Work out the finished part from the listing and answer in its coordinate system (mm). Face numbers are marked on the shaded views. A direction names the side the tool comes from. Coordinates: 2 decimals unless noted, no trailing zeros. Order: outer loops, then holes, each group sorted by start corner. A loop starts at its lowest first (then second) coordinate and runs counter-clockwise, first axis right, second up. Notation, with made-up numbers: (10, -20) -> (55, -20) arc R32 ccw to (55, 17) -> close; hole circle Ø5 at (0, 57.5). An arc over 180 degrees is marked (long way). Answer as CSV lines item,"result". Start each with the question number.
Item 1: Section C-C (x = 10) is taken. Write down the section's boundary in (y, z), then the cut area to 3 significant figures.
Item 2: Which of the six approach directions +Z, -Z, +X, -X, +Y, -Y give full straight-line access (tool end or side, diameter ignored) to the marked faces 4, 5 and 6?
Item 3: Straight lines are drawn through the part: L1, parallel to Z at x = 11.8, y = 0; L2, parallel to Y at x = 2.25, z = 7.75; L3, parallel to Z at x = 8, y = -5. For each, find the intervals that lie inside material, in ascending order.
Item 4: For a pull along X with two mould halves and no side action, classify the marked faces 1, 2 and 3 as pulls with the +X half, pulls with the -X half, needs draft (parallel to the pull), parting line crosses it, or undercut.
Item 5: Section B-B (y = 3.75) is taken. Write down the section's boundary in (x, z), then the cut area to 3 significant figures.
Item 6: Section A-A (x = 0) is taken. Write down the section's boundary in (y, z), then the cut area to 3 significant figures.
Item 7: Each of these flat-tipped pins is pushed along its axis until it touches: pin 1 Ø1.2 at (x, z) = (-1.5, 3) entering from -Y; pin 2 Ø4 at (y, z) = (-7, 4.5) entering from +X; pin 3 Ø3 at (y, z) = (0, 6.75) entering from +X; pin 4 Ø2.5 at (x, y) = (-6.72, -6.72) entering from +Z. Where does it stop, or does it pass through?
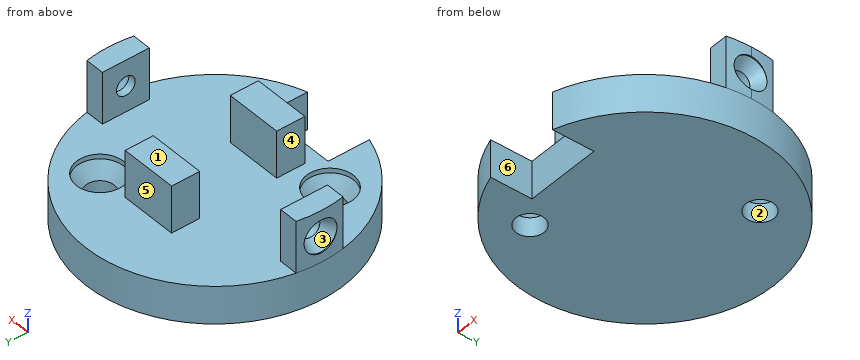
```python
from build123d import *

# Parameters (mm, degrees)
SKETCH1_R           = 13.75
BOSS_EXTRUDE1_DEPTH = 4
BOSS_EXTRUDE2_DEPTH = 5.5
CIRPATTERN1_COUNT   = 2
CIRPATTERN1_ANGLE   = 180
SKETCH10_W          = 2.5
SKETCH10_H          = 0.549822385
CUT_EXTRUDE3_DEPTH  = 21.208290541
BOSS_EXTRUDE4_DEPTH = 5


# Read off the part's stored shape, not the designer's step: Cut-Revolve2
with BuildPart() as part:
    # Sketch1 → Boss-Extrude1 (new body)
    with BuildSketch(Plane.XY):
        Circle(SKETCH1_R)
    extrude(amount=BOSS_EXTRUDE1_DEPTH)

    # Sketch2 → Boss-Extrude2 (add)
    with BuildSketch(Plane.XY.offset(4)):
        with BuildLine():
            Line((-11.520817283, 2.5), (-13.520817283, 2.5))
            ThreePointArc((-13.520817283, 2.5), (-13.75, 0), (-13.520817283, -2.5))
            Line((-13.520817283, -2.5), (-11.520817283, -2.5))
            Line((-11.520817283, -2.5), (-11.520817283, 2.5))
        make_face()
        with BuildLine():
            Line((11.520817283, -2.5), (13.520817283, -2.5))
            ThreePointArc((13.520817283, -2.5), (13.692584446, -1.255241483), (13.75, 0))
            ThreePointArc((13.75, 0), (13.692584446, 1.255241483), (13.520817283, 2.5))
            Line((13.520817283, 2.5), (11.520817283, 2.5))
            Line((11.520817283, 2.5), (11.520817283, -2.5))
        make_face()
    extrude(amount=BOSS_EXTRUDE2_DEPTH)

    # Cut-Revolve2 outline → Cut-Revolve2 (revolve, cut)
    with BuildSketch(Plane.YX.offset(-6.75)):
        Polygon((1.75, -13.750045784), (1.75, -13.638181658), (1, -12.338181697), (1, -11.520817283), (0, -11.520817283), (0, -13.750045784), align=None)
    cut_revolve2 = revolve(axis=Axis((0, 0, 6.75), (1, 0, 0)), mode=Mode.SUBTRACT)

    # CirPattern1: Cut-Revolve2 ×2 about axis
    cirpattern1_axis = Axis((0, 0, 0), (0, 0, 1))
    for i in range(1, CIRPATTERN1_COUNT):
        add(cut_revolve2.rotate(cirpattern1_axis, i * CIRPATTERN1_ANGLE / (CIRPATTERN1_COUNT - 1)), mode=Mode.SUBTRACT)

    # Sketch10 → Cut-Revolve3 (revolve, cut)
    with BuildSketch(Plane(origin=(0, 0, 0), x_dir=(-0.7071067811865561, -0.7071067811865389, 0), z_dir=(-0.7071067811865389, 0.7071067811865561, 0)), mode=Mode.PRIVATE) as cut_revolve3_sk:
        Polygon((-8, 2), (-7, 3.5), (-9.5, 3.5), (-9.5, 0), (-8, 0), align=None)
        with Locations((-8.25, 3.774911193)):
            Rectangle(SKETCH10_W, SKETCH10_H)
    cut_revolve3 = revolve(cut_revolve3_sk.sketch.rotate(Axis((6.717514421, 6.717514421, 0), (0, 0, 1)), 315), axis=Axis((6.717514421, 6.717514421, 0), (0, 0, 1)), mode=Mode.SUBTRACT)

    # Mirror1: Cut-Revolve3 across plane
    add(cut_revolve3.mirror(Plane(origin=(0, 0, 0), x_dir=(0, 0, 1), z_dir=(-0.7071067811865561, -0.7071067811865389, 0))), mode=Mode.SUBTRACT)

    # Sketch11 → Cut-Extrude3 (cut, through all)
    with BuildSketch(Plane.XY.offset(4)):
        with BuildLine():
            ThreePointArc((-4, -13.155322117), (-2.021981816, -13.600517988), (-8e-09, -13.75))
            ThreePointArc((-8e-09, -13.75), (2.021981807, -13.600517989), (4, -13.155322117))
            Line((4, -13.155322117), (4, -8.75))
            Line((4, -8.75), (-4, -8.75))
            Line((-4, -8.75), (-4, -13.155322117))
        make_face()
    extrude(amount=-CUT_EXTRUDE3_DEPTH, mode=Mode.SUBTRACT)

    # Sketch12 → Boss-Extrude4 (add)
    with BuildSketch(Plane.XY.offset(4)):
        Polygon((-3, 7.1), (-3, 4.1), (0, 4.1), (3, 4.1), (3, 7.1), align=None)
        Polygon((0, -4.1), (-3, -4.1), (-3, -7.1), (3, -7.1), (3, -4.1), align=None)
    extrude(amount=BOSS_EXTRUDE4_DEPTH)


solid = part.part
```
Checked values:
1,outline,"(-9.44, 0) -> (9.44, 0) -> (9.44, 4) -> (-9.44, 4) -> close"
1,area,"75.5 mm^2"
2,face 4,"+Z, -X, +Y, -Y"
2,face 5,"+Z, +X, -X, +Y"
2,face 6,"+Z, -Z, -Y"
3,L1,"z = 0 to 5.75, 7.75 to 9.5"
3,L2,"y = -7.1 to -4.1, 4.1 to 7.1"
3,L3,"z = 0 to 4"
4,face 1,"needs draft"
4,face 2,"undercut"
4,face 3,"pulls with the -X half"
5,outline,"(-13.23, 0) -> (13.23, 0) -> (13.23, 4) -> (-13.23, 4) -> close"
5,area,"106 mm^2"
6,outline,"(-8.75, 0) -> (13.75, 0) -> (13.75, 4) -> (7.1, 4) -> (7.1, 9) -> (4.1, 9) -> (4.1, 4) -> (-4.1, 4) -> (-4.1, 9) -> (-7.1, 9) -> (-7.1, 4) -> (-8.75, 4) -> close"
6,area,"120 mm^2"
7,pin 1,"stops at y = -8.75"
7,pin 2,"stops at x = 12.78"
7,pin 3,"stops at x = 13.2"
7,pin 4,"passes through"
